```python
from build123d import *

# Parameters (mm, degrees)
EXTRUDE_1_DEPTH     = 1.2
EXTRUDE_2_DEPTH     = 5
SKETCH_6_R          = 2.5
EXTRUDE_3_DEPTH     = 2
SKETCH_7_R          = 1
CUT_EXTRUDE_1_DEPTH = 113.237393177
SKETCH_8_R          = 2
EXTRUDE_4_DEPTH     = 2.5
CHAMFER_1_SIZE      = 1


with BuildPart() as part:
    # Эскиз4 → Бобышка-Вытянуть1 (new body)
    with BuildSketch(Plane.XY):
        with BuildLine():
            Line((71.69999924, 81.74999906), (71.70000051, 2.500002823))
            ThreePointArc((71.70000051, 2.500002823), (70.909189394, 0.590811786), (68.99999916, -0.20000127))
            Line((68.99999916, -0.20000127), (2.50000008, -0.20000127))
            ThreePointArc((2.50000008, -0.20000127), (0.590809846, 0.590811786), (-0.20000127, 2.500002823))
            Line((-0.20000127, 2.500002823), (-0.2, 81.74999906))
            ThreePointArc((-0.2, 81.74999906), (0.590811714, 83.659187426), (2.50000008, 84.44999914))
            Line((2.50000008, 84.44999914), (68.99999916, 84.44999914))
            ThreePointArc((68.99999916, 84.44999914), (70.909187526, 83.659187426), (71.69999924, 81.74999906))
        make_face()
    extrude(amount=EXTRUDE_1_DEPTH)

    # Эскиз5 → Бобышка-Вытянуть2 (add)
    with BuildSketch(Plane.XY):
        with BuildLine():
            Line((-1.2, 81.74999906), (-1.20000127, 2.500002839))
            ThreePointArc((-1.20000127, 2.500002839), (-0.116296941, -0.116294989), (2.50000008, -1.20000127))
            Line((2.50000008, -1.20000127), (68.99999916, -1.20000127))
            ThreePointArc((68.99999916, -1.20000127), (71.616296534, -0.116294636), (72.70000051, 2.500003839))
            Line((72.70000051, 2.500003839), (72.69999924, 81.749999076))
            ThreePointArc((72.69999924, 81.749999076), (71.616294301, 84.366294213), (68.99999916, 85.44999914))
            Line((68.99999916, 85.44999914), (2.50000008, 85.44999914))
            ThreePointArc((2.50000008, 85.44999914), (-0.116295067, 84.366294207), (-1.2, 81.74999906))
        make_face()
        with BuildLine():
            Line((-0.2, 81.74999906), (-0.20000127, 2.500002823))
            ThreePointArc((-0.20000127, 2.500002823), (0.590809846, 0.590811786), (2.50000008, -0.20000127))
            Line((2.50000008, -0.20000127), (68.99999916, -0.20000127))
            ThreePointArc((68.99999916, -0.20000127), (70.909189394, 0.590811786), (71.70000051, 2.500002823))
            Line((71.70000051, 2.500002823), (71.69999924, 81.74999906))
            ThreePointArc((71.69999924, 81.74999906), (70.909187526, 83.659187426), (68.99999916, 84.44999914))
            Line((68.99999916, 84.44999914), (2.50000008, 84.44999914))
            ThreePointArc((2.50000008, 84.44999914), (0.590811714, 83.659187426), (-0.2, 81.74999906))
        make_face(mode=Mode.SUBTRACT)
    extrude(amount=EXTRUDE_2_DEPTH)

    # Эскиз6 → Бобышка-Вытянуть3 (add)
    with BuildSketch(Plane.XY.offset(1.2)):
        with Locations((48.25000002, 47.49999898)):
            Circle(SKETCH_6_R)
        with BuildLine():
            Line((2.50000008, 84.44999914), (5.226059178, 84.44999914))
            Line((5.226059178, 84.44999914), (5.226059178, 81.007828318))
            ThreePointArc((5.226059178, 81.007828318), (4.493826131, 79.240061365), (2.726059178, 78.507828318))
            Line((2.726059178, 78.507828318), (-0.200000052, 78.507828318))
            Line((-0.200000052, 78.507828318), (-0.2, 81.74999906))
            ThreePointArc((-0.2, 81.74999906), (0.590811714, 83.659187426), (2.50000008, 84.44999914))
        make_face()
        with BuildLine():
            Line((-0.20000127, 2.500002823), (-0.200001232, 4.890114712))
            Line((-0.200001232, 4.890114712), (2.403331994, 4.890114712))
            ThreePointArc((2.403331994, 4.890114712), (4.171098947, 4.157881665), (4.903331994, 2.390114712))
            Line((4.903331994, 2.390114712), (4.903331994, -0.20000127))
            Line((4.903331994, -0.20000127), (2.50000008, -0.20000127))
            ThreePointArc((2.50000008, -0.20000127), (0.590809846, 0.590811786), (-0.20000127, 2.500002823))
        make_face()
        with BuildLine():
            Line((-0.200000511, 49.872119205), (2.726059178, 49.872119205))
            ThreePointArc((2.726059178, 49.872119205), (4.493826131, 49.139886157), (5.226059178, 47.372119205))
            Line((5.226059178, 47.372119205), (5.226059178, 41.864390239))
            ThreePointArc((5.226059178, 41.864390239), (4.493826131, 40.096623286), (2.726059178, 39.364390239))
            Line((2.726059178, 39.364390239), (-0.200000511, 39.364390239))
            Line((-0.200000511, 39.364390239), (-0.200000511, 49.872119205))
        make_face()
        with BuildLine():
            Line((68.99999916, -0.20000127), (66.469541981, -0.20000127))
            Line((66.469541981, -0.20000127), (66.469541981, 2.390114712))
            ThreePointArc((66.469541981, 2.390114712), (67.201775029, 4.157881665), (68.969541981, 4.890114712))
            Line((68.969541981, 4.890114712), (71.700000472, 4.890114712))
            Line((71.700000472, 4.890114712), (71.70000051, 2.500002823))
            ThreePointArc((71.70000051, 2.500002823), (70.909189394, 0.590811786), (68.99999916, -0.20000127))
        make_face()
        with BuildLine():
            Line((45.035976698, 84.44999914), (51.177915607, 84.44999914))
            Line((51.177915607, 84.44999914), (51.177915607, 80.986834439))
            ThreePointArc((51.177915607, 80.986834439), (50.44568256, 79.219067486), (48.677915607, 78.486834439))
            Line((48.677915607, 78.486834439), (47.535976698, 78.486834439))
            ThreePointArc((47.535976698, 78.486834439), (45.768209745, 79.219067486), (45.035976698, 80.986834439))
            Line((45.035976698, 80.986834439), (45.035976698, 84.44999914))
        make_face()
        with BuildLine():
            Line((71.699999835, 44.598653312), (68.631763305, 44.598653312))
            ThreePointArc((68.631763305, 44.598653312), (66.863996352, 43.866420264), (66.131763305, 42.098653312))
            Line((66.131763305, 42.098653312), (66.131763305, 41.579341714))
            ThreePointArc((66.131763305, 41.579341714), (66.863996352, 39.811574761), (68.631763305, 39.079341714))
            Line((68.631763305, 39.079341714), (71.699999835, 39.079341714))
            Line((71.699999835, 39.079341714), (71.699999835, 44.598653312))
        make_face()
    extrude(amount=EXTRUDE_3_DEPTH)

    # Эскиз7 → Вырез-Вытянуть1 (cut, through all)
    with BuildSketch(Plane.XY.offset(3.2)):
        with Locations((2.74999958, 81.49999956)):
            Circle(SKETCH_7_R)
        with Locations((48.25000002, 81.49999956)):
            Circle(SKETCH_7_R)
        with Locations((48.25000002, 47.49999898)):
            Circle(SKETCH_7_R)
        with Locations((68.99999916, 41.99999982)):
            Circle(SKETCH_7_R)
        with Locations((2.74999958, 47.49999898)):
            Circle(SKETCH_7_R)
        with Locations((2.50000008, 41.99999982)):
            Circle(SKETCH_7_R)
        with Locations((2.50000008, 2.50000008)):
            Circle(SKETCH_7_R)
        with Locations((68.99999916, 2.50000008)):
            Circle(SKETCH_7_R)
    extrude(amount=-CUT_EXTRUDE_1_DEPTH, mode=Mode.SUBTRACT)

    # Эскиз8 → Бобышка-Вытянуть4 (add)
    # profile 1 of 2: a face of its own
    with BuildSketch(Plane.XY):
        with BuildLine():
            Line((-5.700000635, 46.12500095), (-1.200000571, 46.12500095))
            Line((-1.200000571, 46.12500095), (-1.200000699, 38.12500095))
            Line((-1.200000699, 38.12500095), (-5.700000635, 38.12500095))
            ThreePointArc((-5.700000635, 38.12500095), (-9.700000635, 42.12500095), (-5.700000635, 46.12500095))
        make_face()
        with Locations((-5.700000635, 42.12500095)):
            Circle(SKETCH_8_R, mode=Mode.SUBTRACT)
    # profile 2 of 2: a face of its own
    with BuildSketch(Plane.XY):
        with BuildLine():
            Line((72.699999939, 38.12500095), (77.199999875, 38.12500095))
            ThreePointArc((77.199999875, 38.12500095), (81.199999875, 42.12500095), (77.199999875, 46.12500095))
            Line((77.199999875, 46.12500095), (72.699999811, 46.12500095))
            Line((72.699999811, 46.12500095), (72.699999939, 38.12500095))
        make_face()
        with Locations(Location((77.199999875, 42.12500095, 0), (0, 0, 180))):
            Circle(SKETCH_8_R, mode=Mode.SUBTRACT)
    extrude(amount=EXTRUDE_4_DEPTH)

    # Фаска1
    chamfer_1_edges = [part.edges().sort_by_distance(p)[0] for p in [
        (-7.700000635, 42.12500095, 2.5),
        (79.199999875, 42.12500095, 2.5),
    ]]
    chamfer(chamfer_1_edges, length=CHAMFER_1_SIZE)


solid = part.part
```
Geometry check sheet. Reference: the model listing, model coordinates, mm. A direction names the side the tool comes from. Give positions to 0.01 mm unless a question says otherwise; leave off trailing zeros. Write each loop counter-clockwise with the first axis right and the second up, starting at its lowest first coordinate (ties: lowest second). Pieces come first, ordered by that corner, then holes.
1) Section check B-B, the plane x = 57. Record the boundary of the cut face in (y, z), and give its area (3 significant figures).
2) Material ranges on L1, parallel to X at y = 42, z = 0.85; L2, parallel to Y at x = 48.25, z = 1; L3, parallel to X at y = 15.5, z = 4.85, recorded low to high.
3) Release check for a two-part mould opening along X. For faces 4 (the cylindrical face through (47.25, 81.54, 1.62)), 5 (the flat face through (-1.2, 43, 3)), 6 (the flat face through (75, 38.125, 1)) record: pulls with the +X half, pulls with the -X half, needs draft (parallel to the pull), parting line crosses it, or undercut.
4) Section check A-A, the plane y = 55. Record the boundary of the cut face in (x, z).
5) Gauge pin test, flat ends, axial feed: pin 1 (1.7 mm diameter, centred on x = 68, y = 43, fed in from +Z); pin 2 (1.2 mm diameter, centred on x = 2.5, y = 2.5, fed in from +Z); pin 3 (1.6 mm diameter, centred on y = 1.5, z = 1.5, fed in from -X); pin 4 (2 mm diameter, centred on x = 75.5, z = 1.5, fed in from -Y) (3 decimals). Record the tip position at first contact, or that the pin passes through.
6) Access from +Z, -Z, +X, -X, +Y, -Y to the whole of each face (thin tool, end or side, straight path). Record for faces 1 (the flat face through (-3, 38.125, 1)), 2 (the flat face through (1, 49.872, 2)), 3 (the cylindrical face through (2.96, 1.61, 1.62)).
Computed:
1. outline: (-1.2, 0) - (85.45, 0) - (85.45, 5) - (84.45, 5) - (84.45, 1.2) - (-0.2, 1.2) - (-0.2, 5) - (-1.2, 5) - close
1. area: 112 mm2
2. L1: x = -9.7 to -7.7, -3.7 to 1.5, 3.5 to 68, 70 to 75.2, 79.2 to 81.2
2. L2: y = -1.2 to 46.5, 48.5 to 80.5, 82.5 to 85.45
2. L3: x = -1.2 to -0.2, 71.7 to 72.7
3. face 4: undercut
3. face 5: pulls with the -X half
3. face 6: needs draft
4. outline: (-1.2, 0) - (72.7, 0) - (72.7, 5) - (71.7, 5) - (71.7, 1.2) - (-0.2, 1.2) - (-0.2, 5) - (-1.2, 5) - close
5. pin 1: stops at z = 3.2
5. pin 2: passes through
5. pin 3: stops at x = -1.19
5. pin 4: stops at y = 38.125
6. face 1: +Z, -Z, -X, -Y
6. face 2: +Z
6. face 3: +Z, -Z
